Read the model definition and answer for the solid it produces. Units are mm, in the model's axes. Coordinates: 2 decimals unless noted, no trailing zeros. Write each loop counter-clockwise with the first axis right and the second up, starting at its lowest first coordinate (ties: lowest second). Pieces come first, ordered by that corner, then holes.
(1) The part is cut by section A-A, the plane y = 500. Determine the outline of the cut face in (x, z), and give its area (3 significant figures).
(2) The part is cut by section C-C, the plane z = 2. Determine the outline of the cut face in (x, y).
(3) Determine the mould class of faces 1 (the cylindrical face through (182.57, 256.61, 4.93)), 2 (the flat face through (271, 840, 0)) for opening direction X: pulls with the +X half, pulls with the -X half, needs draft (parallel to the pull), parting line crosses it, or undercut.
(4) Straight lines are drawn through the part: line 1 along Y through (x, z) = (500, 4.5); line 2 along X through (y, z) = (337, 7.75); line 3 along Y through (x, z) = (623.5, 6). For each, find the intervals that lie inside material, in ascending order.
(5) Given pin 1 (4 mm diameter, centred on y = 835, z = 7, fed in from -X), flat-ended and moving along its own axis, determine where the tip first touches the part or whether it passes through.
```python
from build123d import *

# Parameters (mm, degrees)
CYLINDER_R     = 400
CYLINDER_DEPTH = 10
BOX_W          = 1000
BOX_H          = 1000
BOX_DEPTH      = 10


with BuildPart() as cylinder:
    # Cylinder → Cylinder (new body)
    with BuildSketch(Plane(origin=(500, 500, 0), x_dir=(1, 0, 0), z_dir=(0, 0, 1))):
        Circle(CYLINDER_R)
    extrude(amount=CYLINDER_DEPTH)


with BuildPart() as cut:
    # Box → Box (new body)
    with BuildSketch(Plane.XY):
        with Locations((500, 500)):
            Rectangle(BOX_W, BOX_H)
    extrude(amount=BOX_DEPTH)

    # Cut: cut Cylinder
    add(cylinder.part, mode=Mode.SUBTRACT)


solid = cut.part
```
Computed:
1. outline: (0, 0) - (100, 0) - (100, 10) - (0, 10) - close; (900, 0) - (1000, 0) - (1000, 10) - (900, 10) - close
1. area: 2,000 mm2
2. outline: (0, 0) - (1000, 0) - (1000, 1000) - (0, 1000) - close; hole circle Ø800 at (500, 500)
3. face 1: undercut
3. face 2: needs draft
4. line 1: y = 0 to 100, 900 to 1000
4. line 2: x = 0 to 134.72, 865.28 to 1000
4. line 3: y = 0 to 119.54, 880.46 to 1000
5. pin 1: stops at x = 0
